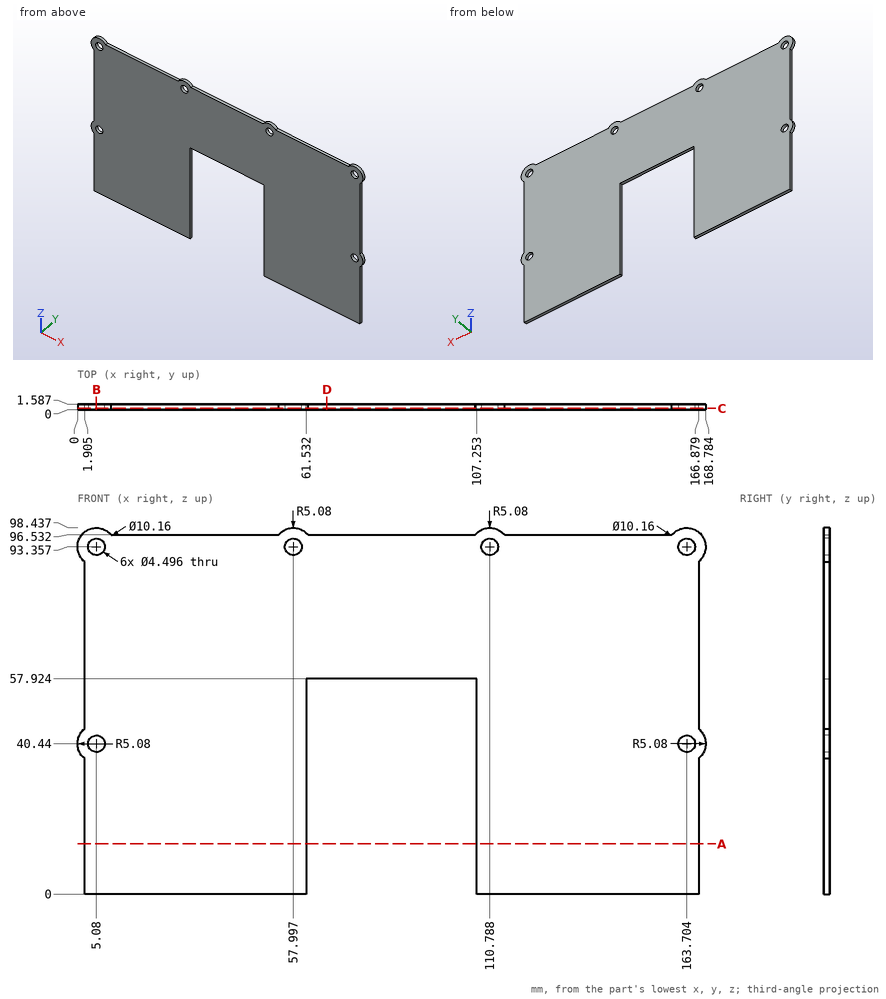
Print and shaded views of the part. All mm, measured from the part's lowest x, y and z. Give positions to 0.01 mm unless a question says otherwise; leave off trailing zeros. Write each loop counter-clockwise with the first axis right and the second up, starting at its lowest first coordinate (ties: lowest second). Pieces come first, ordered by that corner, then holes. Notation, with made-up numbers: (5.5, -7.75) - (40.5, -7.75) arc R19 ccw to (40.5, 7.25) - close; hole circle Ø7 at (19.5, 74.25). An arc over 180 degrees is marked (long way). Put each result on its own line as item: value.
(1) Saw through at D-D (x = 67). List the corners of the cut face in (y, z).
Working result:
outline: (0, 57.92) - (1.59, 57.92) - (1.59, 96.53) - (0, 96.53) - close
(2) Saw through at A-A (z = 13.5). List the corners of the cut face in (x, y) (1 decimal).
Working result:
outline: (1.9, 0) - (61.5, 0) - (61.5, 1.6) - (1.9, 1.6) - close; (107.3, 0) - (166.9, 0) - (166.9, 1.6) - (107.3, 1.6) - close
(3) Saw through at B-B (x = 5.08). List the corners of the cut face in (y, z) (1 decimal).
Working result:
outline: (0, 0) - (1.6, 0) - (1.6, 38.2) - (0, 38.2) - close; (0, 42.7) - (1.6, 42.7) - (1.6, 91.1) - (0, 91.1) - close; (0, 95.6) - (1.6, 95.6) - (1.6, 98.4) - (0, 98.4) - close
(4) Wall check: L1, parallel to Z at x = 5.08, y = 0.85 (1 decimal); L2, parallel to X at y = 0.7, z = 8.5 (1 decimal); L3, parallel to Z at x = 145, y = 1.25. Give the ranges that are in metal, low to high.
Working result:
L1: 0 to 38.2, 42.7 to 91.1, 95.6 to 98.4
L2: 1.9 to 61.5, 107.3 to 166.9
L3: 0 to 96.53
(5) Saw through at C-C (y = 0.4). List the corners of the cut face in (x, z) (1 decimal), then the cut area to 3 significant figures.
Working result:
outline: (1.9, 0) - (61.5, 0) - (61.5, 57.9) - (107.3, 57.9) - (107.3, 0) - (166.9, 0) - (166.9, 36.5) arc R5.1 ccw to (166.9, 44.4) - (166.9, 89.4) arc R5.1 ccw (long way) to (159.7, 96.5) - (114.8, 96.5) arc R5.1 ccw to (106.8, 96.5) - (62, 96.5) arc R5.1 ccw to (54, 96.5) - (9, 96.5) arc R5.1 ccw (long way) to (1.9, 89.4) - (1.9, 44.4) arc R5.1 ccw to (1.9, 36.5) - close; hole circle Ø4.5 at (5.1, 40.4); hole circle Ø4.5 at (5.1, 93.4); hole circle Ø4.5 at (58, 93.4); hole circle Ø4.5 at (110.8, 93.4); hole circle Ø4.5 at (163.7, 40.4); hole circle Ø4.5 at (163.7, 93.4)
area: 13,300 mm^2
(6) Drop flat-ended pins along their axis: pin 1 Ø0.8 at (x, y) = (30.5, 1) entering from +Z; pin 2 Ø0.8 at (y, z) = (0.5, 30) entering from -X (1 decimal). Give the stop position or say it passes through.
Working result:
pin 1: z = 96.53
pin 2: x = 1.9
